Here's how the part is built. I have some questions about the finished solid (model axes, mm). Coordinates: 2 decimals unless noted, no trailing zeros. Write each loop counter-clockwise with the first axis right and the second up, starting at its lowest first coordinate (ties: lowest second). Pieces come first, ordered by that corner, then holes. Notation, with made-up numbers: (74, 21.5) - (117, 21.5) arc R17 ccw to (117, 31.5) - close; hole circle Ø1 at (79, 2.5). An arc over 180 degrees is marked (long way). Answer in a Markdown table with one row per item. Add a question column.
Item 1: Imagine slicing it at A-A (y = -71). Please give me the cut outline in (x, z) (3 decimals).
Item 2: Imagine slicing it at D-D (x = 2.2). State how many separate pieces and enclosed holes the cut face has, plus the area to 3 significant figures.
Item 3: Imagine slicing it at C-C (z = -114.5). Please give me the cut outline in (x, y) (3 decimals).
Item 4: If I drill on probe 1 along Y at (x, z) = (1.9, -36.25) (1 decimal); probe 2 along Y at (x, z) = (1.6, -146.25) (1 decimal); probe 3 along Z at (x, y) = (3.05, -288), over which ranges is the centre line in solid material (lowest first)? Write a range as from..to.
Item 5: I'm going to push flat-ended pins straight in: pin 1 (4 mm diameter, centred on y = -57.86, z = -176.25, fed in from -X); pin 2 (10 mm diameter, centred on y = -235.19, z = -191.25, fed in from -X). Where does each tip first touch, or does it pass through?
Item 6: Imagine slicing it at B-B (z = -20). Please give me the cut outline in (x, y) (3 decimals).
from build123d import *

# Parameters (mm, degrees)
SKETCH1_W           = 212.5
SKETCH1_H           = 339.725
SKETCH1_R           = 3.175
BOSS_EXTRUDE1_DEPTH = 3.175
CUT_EXTRUDE1_DEPTH  = 4.175


with BuildPart() as part:
    # Sketch1 → Boss-Extrude1 (new body)
    with BuildSketch(Plane(origin=(0, 0, 0), x_dir=(0, 0, -1), z_dir=(1, 0, 0))):
        with Locations((106.25, -169.8625)):
            Rectangle(SKETCH1_W, SKETCH1_H)
        with Locations((12.7, -12.7)):
            Circle(SKETCH1_R, mode=Mode.SUBTRACT)
        with Locations((199.8, -12.7)):
            Circle(SKETCH1_R, mode=Mode.SUBTRACT)
        with Locations((66.25, -35.2425)):
            Circle(SKETCH1_R, mode=Mode.SUBTRACT)
        with Locations((146.25, -35.2425)):
            Circle(SKETCH1_R, mode=Mode.SUBTRACT)
        with Locations((176.25, -57.8625)):
            Circle(SKETCH1_R, mode=Mode.SUBTRACT)
        with Locations((36.25, -57.8625)):
            Circle(SKETCH1_R, mode=Mode.SUBTRACT)
        with Locations((191.25, -104.5325)):
            Circle(SKETCH1_R, mode=Mode.SUBTRACT)
        with Locations((36.25, -169.8625)):
            Circle(SKETCH1_R, mode=Mode.SUBTRACT)
        with Locations((191.25, -169.8625)):
            Circle(SKETCH1_R, mode=Mode.SUBTRACT)
        with Locations((36.25, -281.8625)):
            Circle(SKETCH1_R, mode=Mode.SUBTRACT)
        with Locations((66.25, -304.4825)):
            Circle(SKETCH1_R, mode=Mode.SUBTRACT)
        with Locations((12.7, -327.025)):
            Circle(SKETCH1_R, mode=Mode.SUBTRACT)
        with Locations((199.8, -327.025)):
            Circle(SKETCH1_R, mode=Mode.SUBTRACT)
        with Locations((146.25, -304.4825)):
            Circle(SKETCH1_R, mode=Mode.SUBTRACT)
        with Locations((191.25, -235.1925)):
            Circle(SKETCH1_R, mode=Mode.SUBTRACT)
    extrude(amount=BOSS_EXTRUDE1_DEPTH)

    # Sketch2 → Cut-Extrude1 (cut, through all)
    with BuildSketch(Plane(origin=(3.175, 0, 0), x_dir=(0, 0, -1), z_dir=(1, 0, 0))):
        with BuildLine():
            Line((165.85, -88.161695758), (165.85, -251.563304242))
            ThreePointArc((165.85, -251.563304242), (164.516472011, -257.22840036), (160.795934799, -261.703801323))
            Line((160.795934799, -261.703801323), (125.904065201, -288.012271))
            ThreePointArc((125.904065201, -288.012271), (122.183527989, -292.487671963), (120.85, -298.152768081))
            Line((120.85, -298.152768081), (120.85, -314.325))
            ThreePointArc((120.85, -314.325), (117.130256121, -323.305256121), (108.15, -327.025))
            Line((108.15, -327.025), (104.35, -327.025))
            ThreePointArc((104.35, -327.025), (95.369743879, -323.305256121), (91.65, -314.325))
            Line((91.65, -314.325), (91.65, -298.152768081))
            ThreePointArc((91.65, -298.152768081), (90.316472011, -292.487671963), (86.595934799, -288.012271))
            Line((86.595934799, -288.012271), (48.147303392, -259.022002919))
            ThreePointArc((48.147303392, -259.022002919), (44.532850149, -257.119362682), (40.501368593, -256.4625))
            Line((40.501368593, -256.4625), (25.4, -256.4625))
            ThreePointArc((25.4, -256.4625), (16.419743879, -252.742756121), (12.7, -243.7625))
            Line((12.7, -243.7625), (12.7, -207.9625))
            ThreePointArc((12.7, -207.9625), (16.419743879, -198.982243879), (25.4, -195.2625))
            Line((25.4, -195.2625), (48.95, -195.2625))
            ThreePointArc((48.95, -195.2625), (57.930256121, -191.542756121), (61.65, -182.5625))
            Line((61.65, -182.5625), (61.65, -157.1625))
            ThreePointArc((61.65, -157.1625), (57.930256121, -148.182243879), (48.95, -144.4625))
            Line((48.95, -144.4625), (25.4, -144.4625))
            ThreePointArc((25.4, -144.4625), (16.419743879, -140.742756121), (12.7, -131.7625))
            Line((12.7, -131.7625), (12.7, -95.9625))
            ThreePointArc((12.7, -95.9625), (16.419743879, -86.982243879), (25.4, -83.2625))
            Line((25.4, -83.2625), (40.501368593, -83.2625))
            ThreePointArc((40.501368593, -83.2625), (44.532850149, -82.605637318), (48.147303392, -80.702997081))
            Line((48.147303392, -80.702997081), (86.595934799, -51.712729))
            ThreePointArc((86.595934799, -51.712729), (90.316472011, -47.237328037), (91.65, -41.572231919))
            Line((91.65, -41.572231919), (91.65, -25.4))
            ThreePointArc((91.65, -25.4), (95.369743879, -16.419743879), (104.35, -12.7))
            Line((104.35, -12.7), (108.15, -12.7))
            ThreePointArc((108.15, -12.7), (117.130256121, -16.419743879), (120.85, -25.4))
            Line((120.85, -25.4), (120.85, -41.572231919))
            ThreePointArc((120.85, -41.572231919), (122.183527989, -47.237328037), (125.904065201, -51.712729))
            Line((125.904065201, -51.712729), (160.795934799, -78.021198677))
            ThreePointArc((160.795934799, -78.021198677), (164.516472011, -82.49659964), (165.85, -88.161695758))
        make_face()
    extrude(amount=-CUT_EXTRUDE1_DEPTH, mode=Mode.SUBTRACT)


solid = part.part
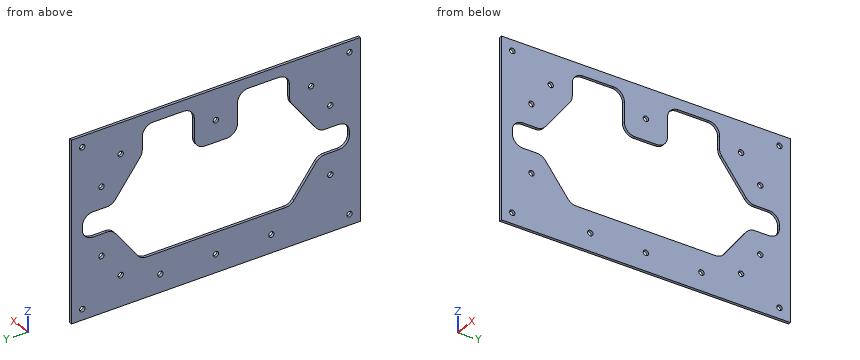
Here are the results:
| question | item | result |
|---|---|---|
| 1 | outline | (0, -212.5) - (3.175, -212.5) - (3.175, -151.484) - (0, -151.484) - close; (0, -61.016) - (3.175, -61.016) - (3.175, 0) - (0, 0) - close |
| 2 | separate pieces | 1 |
| 2 | enclosed holes | 16 |
| 2 | area | 40,400 mm2 |
| 3 | outline | (0, -339.725) - (3.175, -339.725) - (3.175, -325.324) - (0, -325.324) - close; (0, -14.401) - (3.175, -14.401) - (3.175, 0) - (0, 0) - close |
| 4 | probe 1 | y = -339.7..-285, -278.7..-256.5, -195.3..-173, -166.7..-144.5, -83.3..-61, -54.7..0 |
| 4 | probe 2 | y = -339.7..-307.7, -301.3..-272.7, -67.1..-38.4, -32.1..0 |
| 4 | probe 3 | z = -212.5..-125.92, -86.58..0 |
| 5 | pin 1 | passes through |
| 5 | pin 2 | stops at x = 0 |
| 6 | outline | (0, -339.725) - (3.175, -339.725) - (3.175, -255.257) - (0, -255.257) - close; (0, -196.468) - (3.175, -196.468) - (3.175, -143.257) - (0, -143.257) - close; (0, -84.468) - (3.175, -84.468) - (3.175, 0) - (0, 0) - close |
